from build123d import *

# Parameters (mm, degrees)
F0_W     = 75
F0_H     = 75
F1_DEPTH = 100
F2_R     = 7
F3_R     = 32.5
F4_DEPTH = 4
F5_R     = 2.5
F6_DEPTH = 40


with BuildPart() as f1:
    # F0 (on Front) → F1 (new body)
    with BuildSketch(Plane.XZ):
        Rectangle(F0_W, F0_H)
    extrude(amount=-F1_DEPTH)

    # F2
    f2_edges = [f1.edges().sort_by_distance(p)[0] for p in [
        (37.5, 50, 37.5),
        (37.5, 50, -37.5),
        (-37.5, 50, -37.5),
        (-37.5, 50, 37.5),
    ]]
    fillet(f2_edges, radius=F2_R)

    # F3 (on face) → F4 (join)
    with BuildSketch(Plane.XZ):
        Circle(F3_R)
    extrude(amount=F4_DEPTH)

    # F5 (on face) → F6 (join)
    with BuildSketch(Plane.XZ.offset(4)):
        Circle(F5_R)
    extrude(amount=F6_DEPTH)


solid = f1.part
Here's how the part is built. I have some questions about the finished solid (model axes, mm). A direction names the side the tool comes from. Coordinates: 2 decimals unless noted, no trailing zeros. Write each loop counter-clockwise with the first axis right and the second up, starting at its lowest first coordinate (ties: lowest second). Pieces come first, ordered by that corner, then holes. Notation, with made-up numbers: (6.25, -25.75) - (12.25, -25.75) arc R9 ccw to (12.25, -18.75) - close; hole circle Ø11 at (27, -38.5). An arc over 180 degrees is marked (long way). Use one line per item in the form item = value.
1) Suppose I cut it at A-A, the plane x = 0. Write out the boundary of the cut face in (y, z).
Solved:
outline = (-44, -2.5) - (-4, -2.5) - (-4, -32.5) - (0, -32.5) - (0, -37.5) - (100, -37.5) - (100, 37.5) - (0, 37.5) - (0, 32.5) - (-4, 32.5) - (-4, 2.5) - (-44, 2.5) - close
2) On a 3-axis mill with a long thin cutter (end or side, diameter ignored), from which of +Z, -Z, +X, -X, +Y, -Y can I reach the whole of each face in a straight line? I mean faces 1 (the flat face through (-34, 0, 1)), 2 (the flat face through (0, 49, -37.5)). Say none if no direction works.
Solved:
face_1 = -Y
face_2 = -Z, +X, -X, +Y, -Y
3) Suppose I cut it at B-B, the plane z = 0. Write out the boundary of the cut face in (x, y), plus the area to 3 significant figures.
Solved:
outline = (-37.5, 0) - (-32.5, 0) - (-32.5, -4) - (-2.5, -4) - (-2.5, -44) - (2.5, -44) - (2.5, -4) - (32.5, -4) - (32.5, 0) - (37.5, 0) - (37.5, 100) - (-37.5, 100) - close
area = 7,960 mm2
4) Suppose I cut it at C-C, the plane y = -27. Write out the boundary of the cut face in (x, z), plus the area to 3 significant figures.
Solved:
outline = circle Ø5 at (0, 0)
area = 19.6 mm2
5) Suppose I cut it at D-D, the plane x = 21. Write out the boundary of the cut face in (y, z).
Solved:
outline = (-4, -24.8) - (0, -24.8) - (0, -37.5) - (100, -37.5) - (100, 37.5) - (0, 37.5) - (0, 24.8) - (-4, 24.8) - close
6) I need wall thicknesses on line 1 (X direction, y = 47.5, z = -31); line 2 (Y direction, x = -27.5, z = -21); line 3 (Y direction, x = -5.5, z = 15.5). Which ranges of each line are inside material? Lowest first, please.
Solved:
line_1 = -37.48 to 37.48
line_2 = 0 to 100
line_3 = -4 to 100
7) I'm going to push a flat-ended pin straight in: P1, Ø6, axis at x = -5, z = -11, coming from the -Y side. Where does the tip first touch, or does it pass through?
Solved:
P1 = -4
